```python
from build123d import *

# Parameters (mm, degrees)
CUT_EXTRUDE2_DEPTH = 2
FILLET1_R          = 2
CUT_EXTRUDE3_DEPTH = 2
FILLET2_R          = 2
SKETCH7_R          = 2.5
CUT_EXTRUDE4_DEPTH = 34.797190672


with BuildPart() as part:
    # Sketch1 → Revolve1 (revolve)
    with BuildSketch(Plane.XY, mode=Mode.PRIVATE) as revolve1_sk:
        Polygon((0, 0), (-1, 0), (-1, 12.5), (2, 12.5), (2, 10.5), (4, 10.5), (4, 12.5), (6, 12.5), (6, 10.5), (8, 10.5), (8, 12.5), (19, 12.5), (19, 9.5), (-0.010152284, 9.5), align=None)
    revolve(revolve1_sk.sketch.rotate(Axis((0, 0, 0), (-1, 0, 0)), 90), axis=Axis((0, 0, 0), (-1, 0, 0)))

    # Sketch4 → Cut-Extrude2 (cut)
    with BuildSketch(Plane(origin=(0, 12.5, 0), x_dir=(1, 0, 0), z_dir=(0, 1, 0))):
        with BuildLine():
            Line((21.034766018, -5), (21.034766018, 5))
            Line((21.034766018, 5), (12.203400087, 5))
            ThreePointArc((12.203400087, 5), (11.59564841, 0), (12.203400087, -5))
            Line((12.203400087, -5), (21.034766018, -5))
        make_face()
    extrude(amount=-CUT_EXTRUDE2_DEPTH, mode=Mode.SUBTRACT)

    # Fillet1
    # the kernel refuses this fillet: 2 mm, written as the material it adds along each edge
    with BuildSketch(Plane(origin=(32.467135125, 10.5, 0), x_dir=(-0.8863085047711677, 0, -0.46309527569421044), z_dir=(0.46309527569421044, 0, -0.8863085047711677))) as fillet1_piece_1_section:
        with BuildLine():
            CenterArc((20.871486715 - FILLET1_R, FILLET1_R), FILLET1_R, 270, 90)
            Line((20.871486715, FILLET1_R), (20.871486715, 0))
            Line((20.871486715, 0), (20.871486715 - FILLET1_R, 0))
        make_face()
    fillet1_piece_1 = revolve(axis=Axis((32.467135125, 10.5, 0), (0, 1, 0)), revolution_arc=55.174042112, mode=Mode.PRIVATE)
    fillet1_piece_1 = fillet1_piece_1 & Plane(origin=(12.25218062, 0, 0), x_dir=(0, 0, -1), z_dir=(1, 0, 0)) * Cylinder(12.5, 84, mode=Mode.PRIVATE)
    add(fillet1_piece_1)

    # Sketch6 → Cut-Extrude3 (cut)
    with BuildSketch(Plane(origin=(0, -12.5, 0), x_dir=(1, 0, 0), z_dir=(0, 1, 0))):
        with BuildLine():
            Line((19, -5), (12.506184944, -5))
            ThreePointArc((12.506184944, -5), (11.59564841, 0), (12.506184944, 5))
            Line((12.506184944, 5), (19, 5))
            Line((19, 5), (19, -5))
        make_face()
    extrude(amount=CUT_EXTRUDE3_DEPTH, mode=Mode.SUBTRACT)

    # Fillet2
    # the kernel refuses this fillet: 2 mm, written as the material it adds along each edge
    with BuildSketch(Plane(origin=(25.779086317, -10.5, 0), x_dir=(-0.7565204646440288, 0, 0.6539700196299391), z_dir=(0.6539700196299391, 0, 0.7565204646440288))) as fillet2_piece_1_section:
        with BuildLine():
            CenterArc((14.183437907 - FILLET2_R, FILLET2_R), FILLET2_R, 270, 90)
            Line((14.183437907, FILLET2_R), (14.183437907, 0))
            Line((14.183437907, 0), (14.183437907 - FILLET2_R, 0))
        make_face()
    fillet2_piece_1 = revolve(axis=Axis((25.779086317, -10.5, 0), (0, -1, 0)), revolution_arc=81.683194908, mode=Mode.PRIVATE)
    fillet2_piece_1 = fillet2_piece_1 & Plane(origin=(12.166922866, 0, 0), x_dir=(0, 0, -1), z_dir=(1, 0, 0)) * Cylinder(12.5, 57, mode=Mode.PRIVATE)
    add(fillet2_piece_1)

    # Sketch7 → Cut-Extrude4 (cut, through all)
    with BuildSketch(Plane(origin=(0, -12.5, 0), x_dir=(1, 0, 0), z_dir=(0, 1, 0))):
        with Locations(Location((16, 0, 0), (0, 0, 90))):
            Circle(SKETCH7_R)
    extrude(amount=CUT_EXTRUDE4_DEPTH, mode=Mode.SUBTRACT)


solid = part.part
```
Source: CAD feature listing. Evaluate the final solid. Frame: model axes, mm. A direction names the side the tool comes from. Round coordinates to 2 decimals unless told otherwise and drop trailing zeros. Loops run counter-clockwise (first coordinate to the right, second up) from the corner with the lowest first, then second, coordinate; pieces in that order, holes last. Notation, with made-up numbers: M 86,-5 L 117,-5 A33 cw 117,23 Z; hole C 79,9 d7. An arc over 180 degrees is marked long. Use a Markdown table: item, result. Add a question column.
1. Cut plane A-A, the plane x = 16. Output: boundary loops of the cut face in (y, z).
2. Cut plane D-D, the plane x = 1.5. Output: boundary loops of the cut face in (y, z).
3. Ray query, line 1 along Y through (x, z) = (5.75, 0); line 2 along Y through (x, z) = (6.75, 0); line 3 along X through (y, z) = (9.85, 0). Return the intervals inside material, ascending. Write a range as [from, to].
4. Contact query for flat-ended pins moving along their axis: pin 1 (12 mm diameter, centred on y = 2, z = 6.5, fed in from +X); pin 2 (1.5 mm diameter, centred on x = 11.5, z = 8, fed in from +Y); pin 3 (4.5 mm diameter, centred on x = 17.5, z = 2.5, fed in from +Y); pin 4 (0.8 mm diameter, centred on x = 15.5, y = 11, fed in from +Z). Output: stop coordinate, or through.
5. Cut plane B-B, the plane y = -10. Output: boundary loops of the cut face in (x, z), and give its area (3 significant figures).
6. Cut plane C-C, the plane z = 1.25. State how many separate pieces and enclosed holes the cut face has, and give its area (3 significant figures).
7. Set-up query: faces 1 (the flat face through (16, 11, -5)), 2 (the cylindrical face through (16.96, 9.97, -2.31)), 3 (the conical face through (0, 0, 0)), 4 (the flat face through (16, -11, -5)), 5 (the cylindrical face through (3, -3.2, -10)). Return all of +Z, -Z, +X, -X, +Y, -Y with unobstructed straight access to the full face (end or side cutting, diameter ignored); none if empty.
8. Pull-direction query (Z, two-part tool) for faces 6 (the flat face through (16, 11, 5)), 7 (the flat face through (-1, 0, 0)), 8 (the cylindrical face through (7, -3.2, -10)); classes: +Z half, -Z half, draft (parallel to the pull), parting line (faces both ways), or undercut.
Solution:
| question | item | result |
|---|---|---|
| 1 | outline | M -11.46,-5 A12.5 ccw 11.46,-5 L 10.5,-5 L 10.5,-2.5 L 9.17,-2.5 A9.5 cw -9.17,-2.5 L -10.5,-2.5 L -10.5,-5 Z; M -11.46,5 L -10.5,5 L -10.5,2.5 L -9.17,2.5 A9.5 cw 9.17,2.5 L 10.5,2.5 L 10.5,5 L 11.46,5 A12.5 ccw Z |
| 2 | outline | C 0,0 d25; hole C 0,0 d19 |
| 3 | line 1 | y = [-12.5, -9.5], [9.5, 12.5] |
| 3 | line 2 | y = [-10.5, -9.5], [9.5, 10.5] |
| 3 | line 3 | x = [-1, 13.5], [18.5, 19] |
| 4 | pin 1 | stops at x = 19 |
| 4 | pin 2 | stops at y = 10.18 |
| 4 | pin 3 | stops at y = 10.5 |
| 4 | pin 4 | stops at z = 6.62 |
| 5 | outline | M -1,-7.5 L 2,-7.5 L 2,-3.2 L 4,-3.2 L 4,-7.5 L 6,-7.5 L 6,-3.2 L 8,-3.2 L 8,-7.5 L 19,-7.5 L 19,7.5 L 8,7.5 L 8,3.2 L 6,3.2 L 6,7.5 L 4,7.5 L 4,3.2 L 2,3.2 L 2,7.5 L -1,7.5 Z; hole C 16,0 d5 |
| 5 | area | 246 mm2 |
| 6 | separate pieces | 3 |
| 6 | enclosed holes | 0 |
| 6 | area | 87.3 mm2 |
| 7 | face 1 | +X, +Y |
| 7 | face 2 | +Y, -Y |
| 7 | face 3 | +X |
| 7 | face 4 | +X, -Y |
| 7 | face 5 | none |
| 8 | face 6 | undercut |
| 8 | face 7 | draft |
| 8 | face 8 | parting line |
